```python
from build123d import *

# Parameters (mm, degrees)
SKETCH1_R           = 7.540625
BOSS_EXTRUDE1_DEPTH = 6.35
BOSS_EXTRUDE2_START = -6.35
BOSS_EXTRUDE2_DEPTH = 6.35
CIRPATTERN1_COUNT   = 12


with BuildPart() as part:
    # Sketch1 → Boss-Extrude1 (new body)
    with BuildSketch(Plane.XY):
        Circle(SKETCH1_R)
    extrude(amount=BOSS_EXTRUDE1_DEPTH)

    # Sketch2 → Boss-Extrude2 (add)
    with BuildSketch(Plane.XY.offset(6.35).offset(BOSS_EXTRUDE2_START)):
        with BuildLine():
            ThreePointArc((2.408682376, 7.145577276), (1.918658971, 7.606631761), (1.833740268, 8.274076882))
            Line((1.833740268, 8.274076882), (1.867871498, 8.428081478))
            add(Edge.make_bspline(
                [(1.867871498, 8.428081478), (1.890027, 8.589642819), (1.874125743, 8.904843151), (1.802963997, 9.264708669), (1.59380668, 10.019577882), (1.295108843, 10.591204175), (0.97244699, 11.069869155)],
                knots=[0, 0, 0, 0, 0.17205105, 0.330899491, 0.387189732, 1, 1, 1, 1], degree=3))
            ThreePointArc((0.97244699, 11.069869155), (0.703237725, 11.09022601), (0.433613377, 11.10403691))
            add(Edge.make_bspline(
                [(-0.788332001, 8.596512897), (-0.789902704, 8.75957873), (-0.734314822, 9.070245894), (-0.61826726, 9.41824036), (-0.315435205, 10.140644028), (0.053074174, 10.669962321), (0.433613377, 11.10403691)],
                knots=[0, 0, 0, 0, 0.17205105, 0.330899491, 0.387189732, 1, 1, 1, 1], degree=3))
            Line((-0.788332001, 8.596512897), (-0.773926973, 8.439430589))
            ThreePointArc((-0.773926973, 8.439430589), (-0.942472693, 7.788057795), (-1.48680851, 7.392592633))
            ThreePointArc((-1.48680851, 7.392592633), (0.477197028, 7.525510507), (2.408682376, 7.145577276))
        make_face()
    boss_extrude2 = extrude(amount=BOSS_EXTRUDE2_DEPTH)

    # CirPattern1: Boss-Extrude2 ×12 about axis
    cirpattern1_axis = Axis((0, 0, 6.35), (0, 0, -1))
    for i in range(1, CIRPATTERN1_COUNT):
        add(boss_extrude2.rotate(cirpattern1_axis, i * 360 / CIRPATTERN1_COUNT))


solid = part.part
```
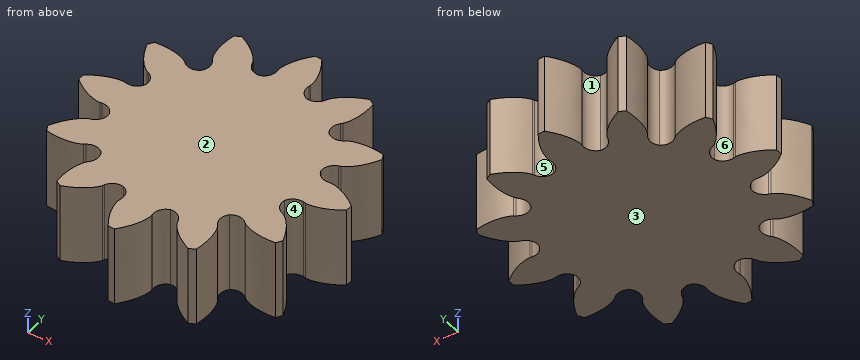
Input: part model. Units: mm. Frame: model coordinates. Face numbers are marked on the shaded views. A direction names the side the tool comes from. Coordinates: 2 decimals unless noted, no trailing zeros.
1) Material intervals for line 1 along X through (y, z) = (7.5, 4.25); line 2 along Y through (x, z) = (9, 4.25); line 3 along Y through (x, z) = (8.75, 3), sorted ascending.
2) Set-up query: the marked faces 1 and 2. Return all of +Z, -Z, +X, -X, +Y, -Y with unobstructed straight access to the full face (end or side cutting, diameter ignored); none if empty.
3) Mould query, pull axis Y, two halves, no side actions, for the marked faces 3, 4, 5 and 6. Classes: pulls with the +Y half, pulls with the -Y half, needs draft (parallel to the pull), parting line crosses it, or undercut.
Check result:
1. line 1: x = -5.16 to -2.06, -1.24 to 1.98, 3.43 to 6.29
1. line 2: y = -6.38 to -4.99, -1.85 to 0.74, 3.15 to 5.29
1. line 3: y = -6.39 to -4.57, -1.88 to 0.78, 2.92 to 5.3
2. face 1: +Z, -Z
2. face 2: +Z, +X, -X, +Y, -Y
3. face 3: needs draft
3. face 4: undercut
3. face 5: pulls with the +Y half
3. face 6: undercut
